```python
from build123d import *

# Parameters (mm, degrees)
SKETCH1_W           = 139.7
SKETCH1_H           = 114.3
BOSS_EXTRUDE1_DEPTH = 12.7
CUT_EXTRUDE2_REACH  = 93.14
SKETCH3_R           = 3.429
SKETCH4_R           = 12.7
CUT_EXTRUDE3_DEPTH  = 7.874


with BuildPart() as part:
    # Sketch1 → Boss-Extrude1 (new body)
    with BuildSketch(Plane(origin=(0, 0, 0), x_dir=(1, 0, 0), z_dir=(0, 1, 0))):
        Rectangle(SKETCH1_W, SKETCH1_H)
    extrude(amount=BOSS_EXTRUDE1_DEPTH)

    # Sketch3 → Cut-Extrude2 (cut, up to next)
    with BuildSketch(Plane.XZ, mode=Mode.PRIVATE) as cut_extrude2_sk1:
        with Locations(Location((-6.35, 44.45, 0), (0, 0, 270))):
            Circle(SKETCH3_R)
    cut_extrude2_tool1 = extrude(cut_extrude2_sk1.sketch, amount=-CUT_EXTRUDE2_REACH, mode=Mode.PRIVATE) & part.part
    # Sketch3 → Cut-Extrude2 (cut, up to next)
    with BuildSketch(Plane.XZ, mode=Mode.PRIVATE) as cut_extrude2_sk2:
        with Locations(Location((-6.35, -44.45, 0), (0, 0, 90))):
            Circle(SKETCH3_R)
    cut_extrude2_tool2 = extrude(cut_extrude2_sk2.sketch, amount=-CUT_EXTRUDE2_REACH, mode=Mode.PRIVATE) & part.part
    # Sketch3 → Cut-Extrude2 (cut, up to next)
    with BuildSketch(Plane.XZ, mode=Mode.PRIVATE) as cut_extrude2_sk3:
        with Locations(Location((57.15, 44.45, 0), (0, 0, 90))):
            Circle(SKETCH3_R)
    cut_extrude2_tool3 = extrude(cut_extrude2_sk3.sketch, amount=-CUT_EXTRUDE2_REACH, mode=Mode.PRIVATE) & part.part
    # Sketch3 → Cut-Extrude2 (cut, up to next)
    with BuildSketch(Plane.XZ, mode=Mode.PRIVATE) as cut_extrude2_sk4:
        with Locations(Location((57.15, -44.45, 0), (0, 0, 270))):
            Circle(SKETCH3_R)
    cut_extrude2_tool4 = extrude(cut_extrude2_sk4.sketch, amount=-CUT_EXTRUDE2_REACH, mode=Mode.PRIVATE) & part.part
    add(cut_extrude2_tool1.solids().sort_by_distance((-6.35, 0, 44.45))[0], mode=Mode.SUBTRACT)
    add(cut_extrude2_tool2.solids().sort_by_distance((-6.35, 0, -44.45))[0], mode=Mode.SUBTRACT)
    add(cut_extrude2_tool3.solids().sort_by_distance((57.15, 0, 44.45))[0], mode=Mode.SUBTRACT)
    add(cut_extrude2_tool4.solids().sort_by_distance((57.15, 0, -44.45))[0], mode=Mode.SUBTRACT)

    # Sketch4 → Cut-Extrude3 (cut)
    with BuildSketch(Plane.XZ):
        with Locations(Location((-53.975, 0, 0), (0, 0, 270))):
            Circle(SKETCH4_R)
    extrude(amount=-CUT_EXTRUDE3_DEPTH, mode=Mode.SUBTRACT)


solid = part.part
```
Check sheet for the modelled part. Datum: model origin and axes. Units: mm. A direction names the side the tool comes from. Round coordinates to 2 decimals unless told otherwise and drop trailing zeros. Loops run counter-clockwise (first coordinate to the right, second up) from the corner with the lowest first, then second, coordinate; pieces in that order, holes last. Notation, with made-up numbers: M -18.5,-15 L -1.5,-15 A15 ccw -1.5,-10 Z; hole C -0.5,60.25 d2. An arc over 180 degrees is marked long. Answer as a JSON object with one key per item and string values.
1. Mould release check, pull along Z, two halves, no side actions. Record for faces 1 (the cylindrical face through (54.259, 6.261, 46.293)), 2 (the flat face through (-1, 0, -1)), 3 (the flat face through (-1, 6, 57.15)): pulls with the +Z half, pulls with the -Z half, needs draft (parallel to the pull), parting line crosses it, or undercut.
Reply:
{"face 1": "undercut", "face 2": "needs draft", "face 3": "pulls with the +Z half"}
2. Section check C-C (y = 2.25). Record the boundary of the cut face in (x, z) (3 decimals).
Reply:
{"outline": "M -69.85,-57.15 L 69.85,-57.15 L 69.85,57.15 L -69.85,57.15 Z; hole C -53.975,0 d25.4; hole C -6.35,-44.45 d6.858; hole C -6.35,44.45 d6.858; hole C 57.15,-44.45 d6.858; hole C 57.15,44.45 d6.858"}
3. Scan lines: line 1 (X direction, y = 4.5, z = 44.45); line 2 (X direction, y = 1, z = 44); line 3 (X direction, y = 6.25, z = 0) (3 decimals). Record each from-to range of solid material in increasing order.
Reply:
{"line 1": "x = -69.85 to -9.78, -2.92 to 53.72, 60.58 to 69.85", "line 2": "x = -69.85 to -9.75, -2.95 to 53.75, 60.55 to 69.85", "line 3": "x = -69.85 to -66.675, -41.275 to 69.85"}
4. Section check D-D (x = -51.5). Record the boundary of the cut face in (y, z), plus the area to 3 significant figures.
Reply:
{"outline": "M 0,-57.15 L 12.7,-57.15 L 12.7,57.15 L 0,57.15 L 0,12.46 L 7.87,12.46 L 7.87,-12.46 L 0,-12.46 Z", "area": "1,260 mm²"}
5. Access from +Z, -Z, +X, -X, +Y, -Y to the whole of each face (thin tool, end or side, straight path). Record for faces 4 (the flat face through (-54, 7.874, 0)), 5 (the flat face through (-1, 12.7, -1)).
Reply:
{"face 4": "-Y", "face 5": "+Z, -Z, +X, -X, +Y"}
6. Gauge pin test, flat ends, axial feed: P1, Ø7.5, axis at x = -51.5, z = 4.5, coming from the -Y side; P2, Ø4, axis at x = 57.15, z = -44.45, coming from the +Y side. Record the tip position at first contact, or that the pin passes through.
Reply:
{"P1": "stops at y = 7.87", "P2": "passes through"}
7. Section check A-A (z = -44.45). Record the boundary of the cut face in (x, y), plus the area to 3 significant figures.
Reply:
{"outline": "M -69.85,0 L -9.78,0 L -9.78,12.7 L -69.85,12.7 Z; M -2.92,0 L 53.72,0 L 53.72,12.7 L -2.92,12.7 Z; M 60.58,0 L 69.85,0 L 69.85,12.7 L 60.58,12.7 Z", "area": "1,600 mm²"}
8. Section check B-B (x = -6.35). Record the boundary of the cut face in (y, z), plus the area to 3 significant figures.
Reply:
{"outline": "M 0,-57.15 L 12.7,-57.15 L 12.7,-47.88 L 0,-47.88 Z; M 0,-41.02 L 12.7,-41.02 L 12.7,41.02 L 0,41.02 Z; M 0,47.88 L 12.7,47.88 L 12.7,57.15 L 0,57.15 Z", "area": "1,280 mm²"}
